```python
from build123d import *

# Parameters (mm, degrees)
CYLINDER_R     = 10
CYLINDER_DEPTH = 60
BOX_W          = 22
BOX_H          = 24
BOX_DEPTH      = 60


with BuildPart() as cilindro:
    # Cylinder → Cylinder (new body)
    with BuildSketch(Plane(origin=(-50, -12, -15), x_dir=(1, 0, 0), z_dir=(0, 0, 1))):
        Circle(CYLINDER_R)
    extrude(amount=CYLINDER_DEPTH)


with BuildPart() as cut:
    # Box → Box (new body)
    with BuildSketch(Plane(origin=(-62, -24, -10), x_dir=(1, 0, 0), z_dir=(0, 0, 1))):
        with Locations((11, 12)):
            Rectangle(BOX_W, BOX_H)
    extrude(amount=BOX_DEPTH)

    # Cut: cut Cilindro
    add(cilindro.part, mode=Mode.SUBTRACT)


solid = cut.part
```
Geometry: final body of the model. Coordinates: model frame, mm. A direction names the side the tool comes from. Round coordinates to 2 decimals unless told otherwise and drop trailing zeros. Use one line per item in the form item = value. Start each with the question number.
Q1. Material intervals for line 1 (Y direction, x = -49.75, z = 16.5); line 2 (Z direction, x = -47, y = -20); line 3 (Y direction, x = -48.5, z = 20), sorted ascending. Write a range as [from, to].
Q2. Access query for faces 1 (the face through (-62, -12, 20)), 2 (the face through (-60, -12, 17)). Directions: +Z, -Z, +X, -X, +Y, -Y. A direction counts if a zero-diameter tool reaches every point of the face in a straight line with its end or side. Return the directions, or none.
Q3. Pin query (flat end, axial travel): pin 1 Ø2 at (x, y) = (-46, -9.5) entering from -Z. Return the tip coordinate at first contact, or that it passes through.
Q4. Mould query, pull axis Y, two halves, no side actions, for faces 3 (the face through (-50, -12, 45)), 4 (the face through (-51, -24, 20)), 5 (the face through (-51, 0, 20)), 6 (the face through (-40, -15, 20)). Classes: +Y half, -Y half, draft (parallel to the pull), parting line (faces both ways), or undercut.
Geometry results:
q1.line_1 = [-24, -22], [-2, 0]
q1.line_2 = [45, 50]
q1.line_3 = [-24, -21.89], [-2.11, 0]
q2.face_1 = +Z, -Z, -X, +Y, -Y
q2.face_2 = -Z
q3.pin_1 = 45
q4.face_3 = undercut
q4.face_4 = -Y half
q4.face_5 = +Y half
q4.face_6 = draft
